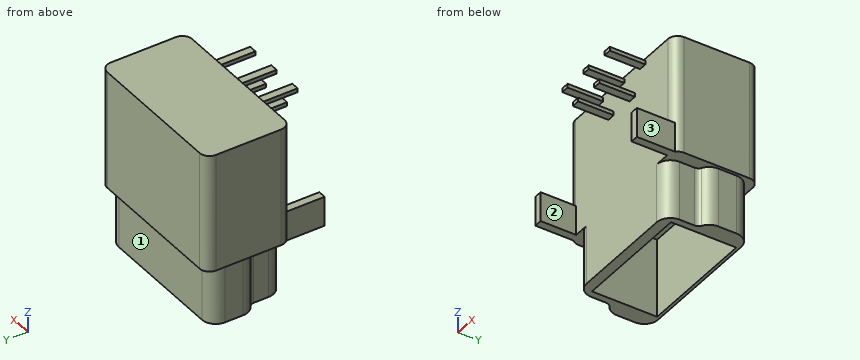
```python
from build123d import *

# Parameters (mm, degrees)
ESQUISSE1_W             = 8
ESQUISSE1_H             = 4.3
EXTRUSION1_DEPTH        = 9
ESQUISSE2_W             = 6
ESQUISSE2_H             = 3.3
ENL_V_MAT_EXTRU_1_DEPTH = 4
ESQUISSE3_W             = 0.4
ESQUISSE3_H             = 1.5
EXTRUSION2_DEPTH        = 1.8
CONG_1_R                = 0.5
ESQUISSE4_W             = 0.4
ESQUISSE4_H             = 0.2
EXTRUSION3_DEPTH        = 1.8
ENL_V_START             = -3
ENL_V_MAT_EXTRU_3_DEPTH = 3


# Read off the part's stored shape, not the designer's step: Enlèv. mat.-Extru.3
with BuildPart() as part:
    # Esquisse1 → Extrusion1 (new body)
    with BuildSketch(Plane.XY):
        with Locations((-4, 2.15)):
            Rectangle(ESQUISSE1_W, ESQUISSE1_H)
    extrude(amount=EXTRUSION1_DEPTH)

    # Esquisse2 → Enlèv. mat.-Extru.1 (cut)
    with BuildSketch(Plane(origin=(0, 0, 0), x_dir=(-1, 0, 0), z_dir=(0, 0, -1))):
        with Locations((4, 2.15)):
            Rectangle(ESQUISSE2_W, ESQUISSE2_H)
    extrude(amount=-ENL_V_MAT_EXTRU_1_DEPTH, mode=Mode.SUBTRACT)

    # Esquisse3 → Extrusion2 (add)
    with BuildSketch(Plane.XZ):
        with Locations((-0.35, 3.75)):
            Rectangle(ESQUISSE3_W, ESQUISSE3_H)
        with Locations((-7.65, 3.75)):
            Rectangle(ESQUISSE3_W, ESQUISSE3_H)
    extrude(amount=EXTRUSION2_DEPTH)

    # Congé1
    # the kernel refuses this fillet: 0.5 mm, written as the material it takes off along each edge
    with BuildSketch(Plane(origin=(0, 0, -1.25), x_dir=(-1, 0, 0), z_dir=(0, 0, 1))) as cong_1_piece_1_section:
        with BuildLine():
            CenterArc((CONG_1_R, -CONG_1_R), CONG_1_R, 90, 90)
            Line((0, -CONG_1_R), (0, 0))
            Line((0, 0), (CONG_1_R, 0))
        make_face()
    cong_1_piece_1 = extrude(amount=11.5, mode=Mode.PRIVATE)
    cong_1_piece_1 = split(cong_1_piece_1, bisect_by=Plane(origin=(-0.251340373, 0.033035409, 3), z_dir=(0, 0, -1)), keep=Keep.TOP, mode=Mode.PRIVATE)
    cong_1_piece_1 = split(cong_1_piece_1, bisect_by=Plane(origin=(-0.15, 0.033035409, 0.875), z_dir=(-1, 0, 0)), keep=Keep.TOP, mode=Mode.PRIVATE)
    add(cong_1_piece_1, mode=Mode.SUBTRACT)
    with BuildSketch(Plane(origin=(0, 0, -1.25), x_dir=(-1, 0, 0), z_dir=(0, 0, 1))) as cong_1_piece_2_section:
        with BuildLine():
            CenterArc((CONG_1_R, -CONG_1_R), CONG_1_R, 90, 90)
            Line((0, -CONG_1_R), (0, 0))
            Line((0, 0), (CONG_1_R, 0))
        make_face()
    cong_1_piece_2 = extrude(amount=11.5, mode=Mode.PRIVATE)
    cong_1_piece_2 = split(cong_1_piece_2, bisect_by=Plane(origin=(-0.054158411, 0.147457064, 3), z_dir=(0, 0, -1)), keep=Keep.TOP, mode=Mode.PRIVATE)
    cong_1_piece_2 = split(cong_1_piece_2, bisect_by=Plane(origin=(-0.15, 0.147457064, 0.875), z_dir=(1, 0, 0)), keep=Keep.TOP, mode=Mode.PRIVATE)
    add(cong_1_piece_2, mode=Mode.SUBTRACT)
    with BuildSketch(Plane(origin=(0, 0, -1.25), x_dir=(-1, 0, 0), z_dir=(0, 0, 1))) as cong_1_piece_3_section:
        with BuildLine():
            CenterArc((CONG_1_R, -CONG_1_R), CONG_1_R, 90, 90)
            Line((0, -CONG_1_R), (0, 0))
            Line((0, 0), (CONG_1_R, 0))
        make_face()
    cong_1_piece_3 = extrude(amount=11.5, mode=Mode.PRIVATE)
    cong_1_piece_3 = split(cong_1_piece_3, bisect_by=Plane(origin=(-0.054158411, 0.147457064, 3), z_dir=(0, 0, 1)), keep=Keep.TOP, mode=Mode.PRIVATE)
    cong_1_piece_3 = split(cong_1_piece_3, bisect_by=Plane(origin=(-0.15, 0.147457064, 3.75), z_dir=(1, 0, 0)), keep=Keep.TOP, mode=Mode.PRIVATE)
    cong_1_piece_3 = split(cong_1_piece_3, bisect_by=Plane(origin=(-0.054158411, 0.147457064, 4.5), z_dir=(0, 0, -1)), keep=Keep.TOP, mode=Mode.PRIVATE)
    add(cong_1_piece_3, mode=Mode.SUBTRACT)
    with BuildSketch(Plane(origin=(0, 0, -1.25), x_dir=(-1, 0, 0), z_dir=(0, 0, 1))) as cong_1_piece_4_section:
        with BuildLine():
            CenterArc((CONG_1_R, -CONG_1_R), CONG_1_R, 90, 90)
            Line((0, -CONG_1_R), (0, 0))
            Line((0, 0), (CONG_1_R, 0))
        make_face()
    cong_1_piece_4 = extrude(amount=11.5, mode=Mode.PRIVATE)
    cong_1_piece_4 = split(cong_1_piece_4, bisect_by=Plane(origin=(-0.15, 0.033035409, 7.375), z_dir=(-1, 0, 0)), keep=Keep.TOP, mode=Mode.PRIVATE)
    cong_1_piece_4 = split(cong_1_piece_4, bisect_by=Plane(origin=(-0.251340373, 0.033035409, 4.5), z_dir=(0, 0, 1)), keep=Keep.TOP, mode=Mode.PRIVATE)
    add(cong_1_piece_4, mode=Mode.SUBTRACT)
    with BuildSketch(Plane(origin=(0, 0, -1.25), x_dir=(-1, 0, 0), z_dir=(0, 0, 1))) as cong_1_piece_5_section:
        with BuildLine():
            CenterArc((CONG_1_R, -CONG_1_R), CONG_1_R, 90, 90)
            Line((0, -CONG_1_R), (0, 0))
            Line((0, 0), (CONG_1_R, 0))
        make_face()
    cong_1_piece_5 = extrude(amount=11.5, mode=Mode.PRIVATE)
    cong_1_piece_5 = split(cong_1_piece_5, bisect_by=Plane(origin=(-0.15, 0.147457064, 7.375), z_dir=(1, 0, 0)), keep=Keep.TOP, mode=Mode.PRIVATE)
    cong_1_piece_5 = split(cong_1_piece_5, bisect_by=Plane(origin=(-0.054158411, 0.147457064, 4.5), z_dir=(0, 0, 1)), keep=Keep.TOP, mode=Mode.PRIVATE)
    add(cong_1_piece_5, mode=Mode.SUBTRACT)
    with BuildSketch(Plane(origin=(-8, 0, -1.25), x_dir=(1, 0, 0), z_dir=(0, 0, 1))) as cong_1_piece_6_section:
        with BuildLine():
            CenterArc((CONG_1_R, CONG_1_R), CONG_1_R, 180, 90)
            Line((0, CONG_1_R), (0, 0))
            Line((0, 0), (CONG_1_R, 0))
        make_face()
    cong_1_piece_6 = extrude(amount=11.5, mode=Mode.PRIVATE)
    cong_1_piece_6 = split(cong_1_piece_6, bisect_by=Plane(origin=(-7.85, 0.033035409, 0.875), z_dir=(1, 0, 0)), keep=Keep.TOP, mode=Mode.PRIVATE)
    cong_1_piece_6 = split(cong_1_piece_6, bisect_by=Plane(origin=(-7.748659627, 0.033035409, 3), z_dir=(0, 0, -1)), keep=Keep.TOP, mode=Mode.PRIVATE)
    add(cong_1_piece_6, mode=Mode.SUBTRACT)
    with BuildSketch(Plane(origin=(-8, 0, -1.25), x_dir=(1, 0, 0), z_dir=(0, 0, 1))) as cong_1_piece_7_section:
        with BuildLine():
            CenterArc((CONG_1_R, CONG_1_R), CONG_1_R, 180, 90)
            Line((0, CONG_1_R), (0, 0))
            Line((0, 0), (CONG_1_R, 0))
        make_face()
    cong_1_piece_7 = extrude(amount=11.5, mode=Mode.PRIVATE)
    cong_1_piece_7 = split(cong_1_piece_7, bisect_by=Plane(origin=(-7.85, 0.147457064, 0.875), z_dir=(-1, 0, 0)), keep=Keep.TOP, mode=Mode.PRIVATE)
    cong_1_piece_7 = split(cong_1_piece_7, bisect_by=Plane(origin=(-7.945841589, 0.147457064, 3), z_dir=(0, 0, -1)), keep=Keep.TOP, mode=Mode.PRIVATE)
    add(cong_1_piece_7, mode=Mode.SUBTRACT)
    with BuildSketch(Plane(origin=(-8, 0, -1.25), x_dir=(1, 0, 0), z_dir=(0, 0, 1))) as cong_1_piece_8_section:
        with BuildLine():
            CenterArc((CONG_1_R, CONG_1_R), CONG_1_R, 180, 90)
            Line((0, CONG_1_R), (0, 0))
            Line((0, 0), (CONG_1_R, 0))
        make_face()
    cong_1_piece_8 = extrude(amount=11.5, mode=Mode.PRIVATE)
    cong_1_piece_8 = split(cong_1_piece_8, bisect_by=Plane(origin=(-7.945841589, 0.147457064, 4.5), z_dir=(0, 0, -1)), keep=Keep.TOP, mode=Mode.PRIVATE)
    cong_1_piece_8 = split(cong_1_piece_8, bisect_by=Plane(origin=(-7.85, 0.147457064, 3.75), z_dir=(-1, 0, 0)), keep=Keep.TOP, mode=Mode.PRIVATE)
    cong_1_piece_8 = split(cong_1_piece_8, bisect_by=Plane(origin=(-7.945841589, 0.147457064, 3), z_dir=(0, 0, 1)), keep=Keep.TOP, mode=Mode.PRIVATE)
    add(cong_1_piece_8, mode=Mode.SUBTRACT)
    with BuildSketch(Plane(origin=(-8, 0, -1.25), x_dir=(1, 0, 0), z_dir=(0, 0, 1))) as cong_1_piece_9_section:
        with BuildLine():
            CenterArc((CONG_1_R, CONG_1_R), CONG_1_R, 180, 90)
            Line((0, CONG_1_R), (0, 0))
            Line((0, 0), (CONG_1_R, 0))
        make_face()
    cong_1_piece_9 = extrude(amount=11.5, mode=Mode.PRIVATE)
    cong_1_piece_9 = split(cong_1_piece_9, bisect_by=Plane(origin=(-7.748659627, 0.033035409, 4.5), z_dir=(0, 0, 1)), keep=Keep.TOP, mode=Mode.PRIVATE)
    cong_1_piece_9 = split(cong_1_piece_9, bisect_by=Plane(origin=(-7.85, 0.033035409, 7.375), z_dir=(1, 0, 0)), keep=Keep.TOP, mode=Mode.PRIVATE)
    add(cong_1_piece_9, mode=Mode.SUBTRACT)
    with BuildSketch(Plane(origin=(-8, 0, -1.25), x_dir=(1, 0, 0), z_dir=(0, 0, 1))) as cong_1_piece_10_section:
        with BuildLine():
            CenterArc((CONG_1_R, CONG_1_R), CONG_1_R, 180, 90)
            Line((0, CONG_1_R), (0, 0))
            Line((0, 0), (CONG_1_R, 0))
        make_face()
    cong_1_piece_10 = extrude(amount=11.5, mode=Mode.PRIVATE)
    cong_1_piece_10 = split(cong_1_piece_10, bisect_by=Plane(origin=(-7.945841589, 0.147457064, 4.5), z_dir=(0, 0, 1)), keep=Keep.TOP, mode=Mode.PRIVATE)
    cong_1_piece_10 = split(cong_1_piece_10, bisect_by=Plane(origin=(-7.85, 0.147457064, 7.375), z_dir=(-1, 0, 0)), keep=Keep.TOP, mode=Mode.PRIVATE)
    add(cong_1_piece_10, mode=Mode.SUBTRACT)
    with BuildSketch(Plane(origin=(-8, 4.3, -1.25), x_dir=(0, -1, 0), z_dir=(0, 0, 1))) as cong_1_piece_11:
        with BuildLine():
            CenterArc((CONG_1_R, CONG_1_R), CONG_1_R, 180, 90)
            Line((0, CONG_1_R), (0, 0))
            Line((0, 0), (CONG_1_R, 0))
        make_face()
    extrude(amount=11.5, mode=Mode.SUBTRACT)
    with BuildSketch(Plane(origin=(0, 4.3, -1.25), x_dir=(0, -1, 0), z_dir=(0, 0, 1))) as cong_1_piece_12:
        with BuildLine():
            CenterArc((CONG_1_R, -CONG_1_R), CONG_1_R, 90, 90)
            Line((0, -CONG_1_R), (0, 0))
            Line((0, 0), (CONG_1_R, 0))
        make_face()
    extrude(amount=11.5, mode=Mode.SUBTRACT)

    # Esquisse4 → Extrusion3 (add)
    with BuildSketch(Plane.XZ):
        with Locations((-2.4, 8.8)):
            Rectangle(ESQUISSE4_W, ESQUISSE4_H)
        with Locations((-5.6, 8.8)):
            Rectangle(ESQUISSE4_W, ESQUISSE4_H)
        with Locations((-4, 8.8)):
            Rectangle(ESQUISSE4_W, ESQUISSE4_H)
        with Locations((-3.2, 7.6)):
            Rectangle(ESQUISSE4_W, ESQUISSE4_H)
        with Locations((-4.8, 7.6)):
            Rectangle(ESQUISSE4_W, ESQUISSE4_H)
    extrude(amount=EXTRUSION3_DEPTH)

    # Enlèv. mat.-Extru.3 outline → Enlèv. mat.-Extru.3 (cut)
    with BuildSketch(Plane(origin=(0, 0, 0), x_dir=(-1, 0, 0), z_dir=(0, 0, -1)).offset(ENL_V_START)):
        with BuildLine():
            Line((0.15, 2.326025404), (0.15, 3.25))
            ThreePointArc((0.15, 3.25), (0.355025253, 3.744974747), (0.85, 3.95))
            Line((0.85, 3.95), (7.15, 3.95))
            ThreePointArc((7.15, 3.95), (7.644974747, 3.744974747), (7.85, 3.25))
            Line((7.85, 3.25), (7.85, 2.326025404))
            ThreePointArc((7.85, 2.326025404), (7.756217783, 1.976025404), (7.5, 1.719807621))
            ThreePointArc((7.5, 1.719807621), (7.390192379, 1.61), (7.35, 1.46))
            Line((7.35, 1.46), (7.35, 0.7))
            ThreePointArc((7.35, 0.7), (7.144974747, 0.205025253), (6.65, 0))
            Line((6.65, 0), (7.5, 0))
            ThreePointArc((7.5, 0), (7.853553391, 0.146446609), (8, 0.5))
            Line((8, 0.5), (8, 3.8))
            ThreePointArc((8, 3.8), (7.853553391, 4.153553391), (7.5, 4.3))
            Line((7.5, 4.3), (0.5, 4.3))
            ThreePointArc((0.5, 4.3), (0.146446609, 4.153553391), (0, 3.8))
            Line((0, 3.8), (0, 0.5))
            ThreePointArc((0, 0.5), (0.146446609, 0.146446609), (0.5, 0))
            Line((0.5, 0), (1.35, 0))
            ThreePointArc((1.35, 0), (0.855025253, 0.205025253), (0.65, 0.7))
            Line((0.65, 0.7), (0.65, 1.46))
            ThreePointArc((0.65, 1.46), (0.609807621, 1.61), (0.5, 1.719807621))
            ThreePointArc((0.5, 1.719807621), (0.243782217, 1.976025404), (0.15, 2.326025404))
        make_face()
    extrude(amount=ENL_V_MAT_EXTRU_3_DEPTH, mode=Mode.SUBTRACT)


solid = part.part
```
Geometry check sheet. Reference: the model listing, model coordinates, mm. Face numbers are marked on the shaded views. A direction names the side the tool comes from. Give positions to 0.01 mm unless a question says otherwise; leave off trailing zeros. Loops run counter-clockwise (first coordinate to the right, second up) from the corner with the lowest first, then second, coordinate; pieces in that order, holes last. Notation, with made-up numbers: M -10,-20.5 L 17,-20.5 A11 cw 17,-3.5 Z; hole C 12,30 d3. An arc over 180 degrees is marked long. Write item = value, one per line.
(1) Tool access check on the marked faces 1, 2 and 3. Record the directions out of +Z, -Z, +X, -X, +Y, -Y that give a thin tool (end or side, any length) a straight path to the whole face; none if there is none.
Answer below:
face_1 = -Z, +X, -X, +Y
face_2 = +Z, -Z, -Y
face_3 = +Z, -Z, +X, -Y
(2) Material ranges on line 1 (X direction, y = -1.5, z = 3.75); line 2 (X direction, y = 1.5, z = 3.25); line 3 (Z direction, x = -5.75, y = 1.25), recorded low to high. Write a range as [from, to].
Answer below:
line_1 = [-7.85, -7.45], [-0.55, -0.15]
line_2 = [-8, -7], [-1, 0]
line_3 = [4, 9]
(3) Sectioned sample at B-B, the plane y = -1. Record the cut outline in (x, z).
Answer below:
outline = M -7.85,3 L -7.45,3 L -7.45,4.5 L -7.85,4.5 Z; M -5.8,8.7 L -5.4,8.7 L -5.4,8.9 L -5.8,8.9 Z; M -5,7.5 L -4.6,7.5 L -4.6,7.7 L -5,7.7 Z; M -4.2,8.7 L -3.8,8.7 L -3.8,8.9 L -4.2,8.9 Z; M -3.4,7.5 L -3,7.5 L -3,7.7 L -3.4,7.7 Z; M -2.6,8.7 L -2.2,8.7 L -2.2,8.9 L -2.6,8.9 Z; M -0.55,3 L -0.15,3 L -0.15,4.5 L -0.55,4.5 Z
(4) Gauge pin test, flat ends, axial feed: pin 1 Ø2.5 at (x, z) = (-3, 1.5) entering from +Y; pin 2 Ø1 at (x, z) = (-3.5, 6) entering from -Y. Record the tip position at first contact, or that the pin passes through.
Answer below:
pin_1 = 3.95
pin_2 = 0
(5) Sectioned sample at D-D, the plane x = -6.25. Record the cut outline in (y, z), plus the area to 4 significant figures.
Answer below:
outline = M 0,0 L 0.5,0 L 0.5,4 L 3.8,4 L 3.8,0 L 3.95,0 L 3.95,3 L 4.3,3 L 4.3,9 L 0,9 Z
area = 24.45 mm2
(6) Sectioned sample at A-A, the plane z = 3.5. Record the cut outline in (x, y), plus the area to 3 significant figures.
Answer below:
outline = M -8,0.5 A0.5 ccw -7.85,0.14 L -7.85,-1.8 L -7.45,-1.8 L -7.45,0 L -0.55,0 L -0.55,-1.8 L -0.15,-1.8 L -0.15,0.14 A0.5 ccw 0,0.5 L 0,3.8 A0.5 ccw -0.5,4.3 L -7.5,4.3 A0.5 ccw -8,3.8 Z; hole M -7,0.5 L -1,0.5 L -1,3.8 L -7,3.8 Z
area = 15.9 mm2
(7) Sectioned sample at C-C, the plane y = 3. Record the cut outline in (x, z), plus the area to 3 significant figures.
Answer below:
outline = M -8,3 L -7.85,3 L -7.85,0 L -7,0 L -7,4 L -1,4 L -1,0 L -0.15,0 L -0.15,3 L 0,3 L 0,9 L -8,9 Z
area = 47.1 mm2
